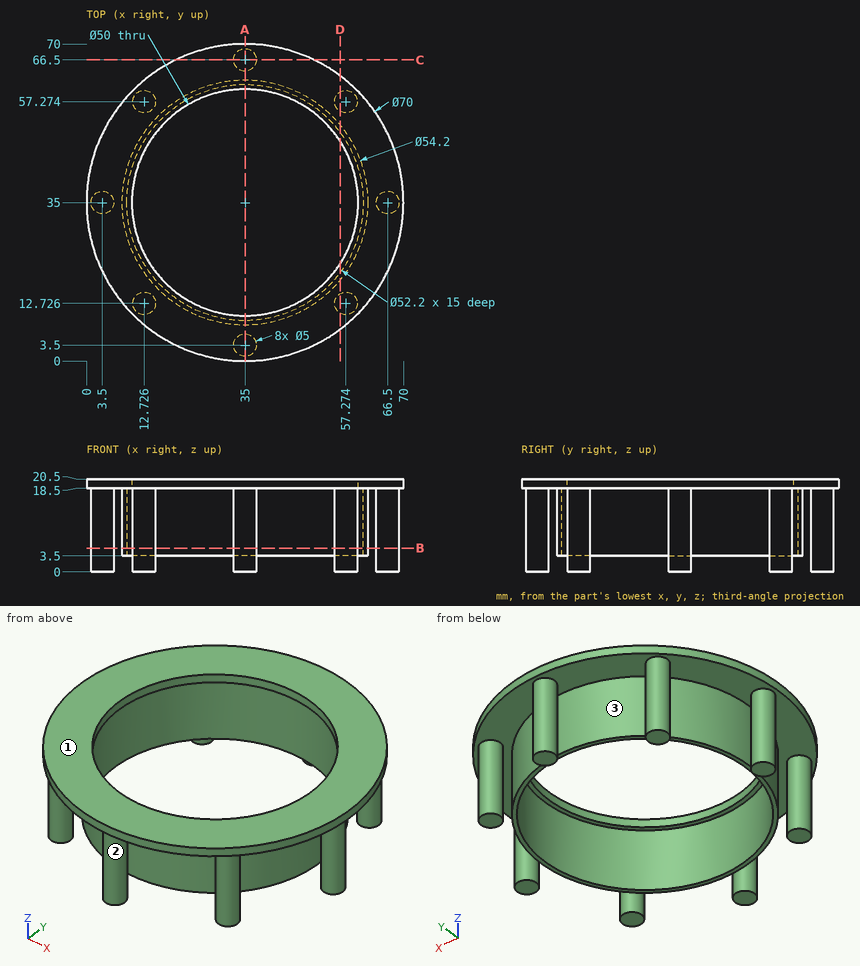
Check sheet for the drawn part. Datum: minimum x, y, z corner. Units: mm. Round coordinates to 2 decimals unless told otherwise and drop trailing zeros. Order: outer loops, then holes, each group sorted by start corner. A loop starts at its lowest first (then second) coordinate and runs counter-clockwise, first axis right, second up. Notation, with made-up numbers: (13, -13.75) - (32, -13.75) arc R16 ccw to (32, 6.25) - close; hole circle Ø7 at (-0.75, 69.5). An arc over 180 degrees is marked (long way). Use a Markdown table: item, result. Add a question column.
(1) Sectioned sample at C-C, the plane y = 66.5. Enter the section's corners in (x, z).
(2) Sectioned sample at D-D, the plane x = 56. Enter the section's corners in (y, z) (1 decimal), and give its area (3 significant figures).
(3) Release check for a two-part mould opening along X. For the marked faces 1, 2 and 3 record: pulls with the +X half, pulls with the -X half, needs draft (parallel to the pull), parting line crosses it, or undercut.
(4) Material ranges on line 1 along Y through (x, z) = (35, 8.5); line 2 along Y through (x, z) = (35, 19); line 3 along Y through (x, z) = (11.5, 4.5) (1 decimal), recorded low to high. Write a range as [from, to].
(5) Sectioned sample at A-A, the plane x = 35. Enter the section's corners in (y, z).
(6) Sectioned sample at B-B, the plane z = 5.25. Count the separate pieces of the cut face and the enclosed holes in it, and give its area (3 significant figures).
(7) Depth check by flat-ended pin: pin 1 (10 mm diameter, centred on x = 54, z = 11.5, fed in from -Y); pin 2 (6 mm diameter, centred on y = 30, z = 16, fed in from +X); pin 3 (10 mm diameter, centred on x = 13, z = 17.5, fed in from +Y). Enter the tip coordinate at first touch or a pass-through.
Answers below:
| question | item | result |
|---|---|---|
| 1 | outline | (19.74, 18.5) - (32.5, 18.5) - (32.5, 0) - (37.5, 0) - (37.5, 18.5) - (50.26, 18.5) - (50.26, 20.5) - (19.74, 20.5) - close |
| 2 | outline | (7, 18.5) - (10.6, 18.5) - (10.6, 0) - (14.9, 0) - (14.9, 18.5) - (17.9, 18.5) - (17.9, 3.5) - (19.5, 3.5) - (19.5, 18.5) - (21.4, 18.5) - (21.4, 20.5) - (7, 20.5) - close; (48.6, 18.5) - (50.5, 18.5) - (50.5, 3.5) - (52.1, 3.5) - (52.1, 18.5) - (55.1, 18.5) - (55.1, 0) - (59.4, 0) - (59.4, 18.5) - (63, 18.5) - (63, 20.5) - (48.6, 20.5) - close |
| 2 | area | 266 mm² |
| 3 | face 1 | needs draft |
| 3 | face 2 | parting line crosses it |
| 3 | face 3 | undercut |
| 4 | line 1 | [1, 6], [7.9, 8.9], [61.1, 62.1], [64, 69] |
| 4 | line 2 | [0, 10], [60, 70] |
| 4 | line 3 | [10.5, 14.9], [21.5, 23.6], [46.4, 48.5], [55.1, 59.5] |
| 5 | outline | (0, 18.5) - (1, 18.5) - (1, 0) - (6, 0) - (6, 18.5) - (7.9, 18.5) - (7.9, 3.5) - (8.9, 3.5) - (8.9, 18.5) - (10, 18.5) - (10, 20.5) - (0, 20.5) - close; (60, 18.5) - (61.1, 18.5) - (61.1, 3.5) - (62.1, 3.5) - (62.1, 18.5) - (64, 18.5) - (64, 0) - (69, 0) - (69, 18.5) - (70, 18.5) - (70, 20.5) - (60, 20.5) - close |
| 6 | separate pieces | 9 |
| 6 | enclosed holes | 1 |
| 6 | area | 324 mm² |
| 7 | pin 1 | y = 10.23 |
| 7 | pin 2 | x = 69.84 |
| 7 | pin 3 | y = 65.54 |
